```python
from build123d import *

# Parameters (mm, degrees)
F0_W     = 114.999984
F0_H     = 15
F0_R     = 3
F0_R_2   = 1.5
F1_DEPTH = 25
F2_R     = 2.5
F3_DEPTH = 25
F2_W     = 103.84956
F2_H     = 15
F4_DEPTH = 5
F5_DEPTH = 10


with BuildPart() as f1:
    # F0 (on Top) → F1 (new body)
    with BuildSketch(Plane.XY):
        with Locations((0, 77.500006)):
            Rectangle(F0_W, F0_H)
        Polygon((-57.499992, 70.000006), (-57.499992, 85.000006), (-67.499992, 85.000006), (-67.499992, -4.999994), (-57.499992, -4.999994), align=None)
        with Locations((-62.5, -6e-06)):
            Circle(F0_R, mode=Mode.SUBTRACT)
        with Locations((-62.500006, 64.999994)):
            Circle(F0_R, mode=Mode.SUBTRACT)
        Polygon((67.499992, 85.000006), (57.499992, 85.000006), (57.499992, 70.000006), (57.499992, -4.999994), (67.499992, -4.999994), align=None)
        with Locations((62.5, 6e-06)):
            Circle(F0_R, mode=Mode.SUBTRACT)
        with Locations((62.499994, 65.000006)):
            Circle(F0_R, mode=Mode.SUBTRACT)
        with Locations((62.499994, 65.000006)):
            Circle(F0_R)
        with Locations((62.499994, 65.000006)):
            Circle(F0_R_2, mode=Mode.SUBTRACT)
        with Locations((62.5, 6e-06)):
            Circle(F0_R)
        with Locations((62.5, 6e-06)):
            Circle(F0_R_2, mode=Mode.SUBTRACT)
        with Locations((-62.5, -6e-06)):
            Circle(F0_R)
        with Locations((-62.5, -6e-06)):
            Circle(F0_R_2, mode=Mode.SUBTRACT)
        with Locations((-62.500006, 64.999994)):
            Circle(F0_R)
        with Locations((-62.500006, 64.999994)):
            Circle(F0_R_2, mode=Mode.SUBTRACT)
    extrude(amount=F1_DEPTH)

    # F2 (on face) → F3 (cut)
    with BuildSketch(Plane.XY.offset(25)):
        with Locations((0, 77.500006)):
            Circle(F2_R)
    extrude(amount=-F3_DEPTH, mode=Mode.SUBTRACT)

    # F2 (on face) → F4 (cut)
    with BuildSketch(Plane.XY.offset(25)):
        with Locations((0.137366, 77.500006)):
            Rectangle(F2_W, F2_H)
        with Locations((0, 77.500006)):
            Circle(F2_R, mode=Mode.SUBTRACT)
    extrude(amount=-F4_DEPTH, mode=Mode.SUBTRACT)

    # F0 (on Top) → F5 (cut)
    with BuildSketch(Plane.XY):
        with Locations((-62.500006, 64.999994)):
            Circle(F0_R)
        with Locations((-62.500006, 64.999994)):
            Circle(F0_R_2, mode=Mode.SUBTRACT)
        with Locations((-62.5, -6e-06)):
            Circle(F0_R)
        with Locations((-62.5, -6e-06)):
            Circle(F0_R_2, mode=Mode.SUBTRACT)
        with Locations((62.5, 6e-06)):
            Circle(F0_R)
        with Locations((62.5, 6e-06)):
            Circle(F0_R_2, mode=Mode.SUBTRACT)
        with Locations((62.499994, 65.000006)):
            Circle(F0_R)
        with Locations((62.499994, 65.000006)):
            Circle(F0_R_2, mode=Mode.SUBTRACT)
    extrude(amount=F5_DEPTH, mode=Mode.SUBTRACT)


solid = f1.part
```
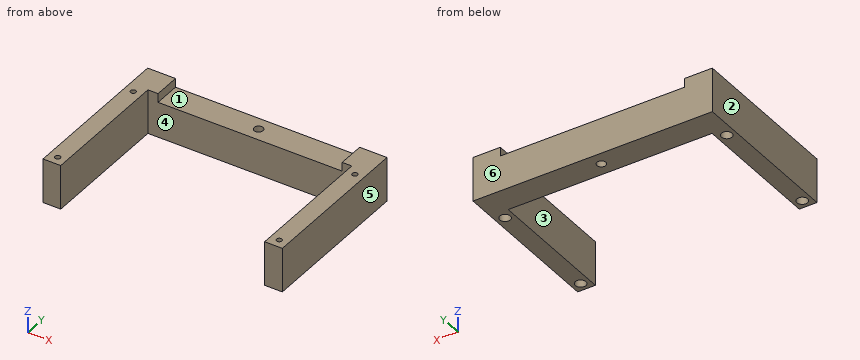
Verification items for the finished model (mm, model axes). Face numbers are marked on the shaded views. A direction names the side the tool comes from. Give positions to 0.01 mm unless a question says otherwise; leave off trailing zeros. Write each loop counter-clockwise with the first axis right and the second up, starting at its lowest first coordinate (ties: lowest second). Pieces come first, ordered by that corner, then holes. Notation, with made-up numbers: (15, 57.5) - (36, 57.5) arc R20 cw to (36, 82.5) - close; hole circle Ø10 at (89.5, 34). An arc over 180 degrees is marked (long way). Put each result on its own line as item: value.
Q1. Section check D-D on x = -62.5. Record the cut outline in (y, z).
Result:
outline: (-5, 0) - (-3, 0) - (-3, 10) - (-1.5, 10) - (-1.5, 25) - (-5, 25) - close; (1.5, 10) - (3, 10) - (3, 0) - (62, 0) - (62, 10) - (63.5, 10) - (63.5, 25) - (1.5, 25) - close; (66.5, 10) - (68, 10) - (68, 0) - (85, 0) - (85, 25) - (66.5, 25) - close
Q2. Section check B-B on x = 0. Record the cut outline in (y, z), and give its area (3 significant figures).
Result:
outline: (70, 0) - (75, 0) - (75, 20) - (70, 20) - close; (80, 0) - (85, 0) - (85, 20) - (80, 20) - close
area: 200 mm2
Q3. Section check C-C on z = 22.25. Record the cut outline in (x, y).
Result:
outline: (-67.5, -5) - (-57.5, -5) - (-57.5, 70) - (-51.79, 70) - (-51.79, 85) - (-67.5, 85) - close; (52.06, 70) - (57.5, 70) - (57.5, -5) - (67.5, -5) - (67.5, 85) - (52.06, 85) - close; hole circle Ø3 at (-62.5, 0); hole circle Ø3 at (-62.5, 65); hole circle Ø3 at (62.5, 0); hole circle Ø3 at (62.5, 65)
Q4. Mould release check, pull along X, two halves, no side actions. Record for the marked faces 4, 5 and 6: released by +X, released by -X, zero draft, split by the parting line, or undercut.
Result:
face 4: undercut
face 5: released by +X
face 6: zero draft
Q5. Set-up check for the marked faces 1, 2 and 3: record each of +Z, -Z, +X, -X, +Y, -Y from which the full face is reachable in a straight line by a thin tool's end or side.
Result:
face 1: +Z, +Y, -Y
face 2: +Z, -Z, -X, +Y, -Y
face 3: +Z, -Z, -Y
Q6. Scan lines: probe 1 along Y at (x, z) = (62.5, 20); probe 2 along Y at (x, z) = (-62.5, 3.25); probe 3 along X at (y, z) = (27, 23). Record each from-to range of solid material in increasing order. Write a range as from..to.
Result:
probe 1: -5..-1.5, 1.5..63.5, 66.5..85
probe 2: -5..-3, 3..62, 68..85
probe 3: -67.5..-57.5, 57.5..67.5
Q7. Section check A-A on y = 56.5. Record the cut outline in (x, z).
Result:
outline: (-67.5, 0) - (-57.5, 0) - (-57.5, 25) - (-67.5, 25) - close; (57.5, 0) - (67.5, 0) - (67.5, 25) - (57.5, 25) - close
Q8. Depth check by flat-ended pin: P1, Ø7.5, axis at x = -1.5, y = 79.5, coming from the +Z side; P2, Ø5.5, axis at x = 62.5, y = 0, coming from the -Z side. Enter the tip coordinate at first touch or a pass-through.
Result:
P1: z = 20
P2: z = 10
